```python
from build123d import *

# Parameters (mm, degrees)
BOSS_EXTRUDE2_DEPTH = 20
SKETCH2_R           = 1.5
CUT_EXTRUDE1_DEPTH  = 30


with BuildPart() as part:
    # Sketch1 → Boss-Extrude2 (new body)
    with BuildSketch(Plane.XY):
        with BuildLine():
            Line((-14, 17.3), (-26.4, 17.3))
            ThreePointArc((-26.4, 17.3), (-29.228427125, 18.471572875), (-30.4, 21.3))
            Line((-30.4, 21.3), (-30.4, 62.205522081))
            Line((-30.4, 62.205522081), (-27.4, 62.205522081))
            Line((-27.4, 62.205522081), (-27.4, 28.3))
            ThreePointArc((-27.4, 28.3), (-26.228427125, 25.471572875), (-23.4, 24.3))
            Line((-23.4, 24.3), (-3, 24.3))
            ThreePointArc((-3, 24.3), (-0.171572875, 23.128427125), (1, 20.3))
            Line((1, 20.3), (1, 9.949874371))
            ThreePointArc((1, 9.949874371), (6.708203932, -7.416198487), (-10, 0))
            Line((-10, 0), (-10, 13.3))
            ThreePointArc((-10, 13.3), (-11.171572875, 16.128427125), (-14, 17.3))
        make_face()
    extrude(amount=BOSS_EXTRUDE2_DEPTH)

    # Sketch2 → Cut-Extrude1 (cut)
    with BuildSketch(Plane.XY.offset(20)):
        Circle(SKETCH2_R)
    extrude(amount=-CUT_EXTRUDE1_DEPTH, mode=Mode.SUBTRACT)


solid = part.part
```
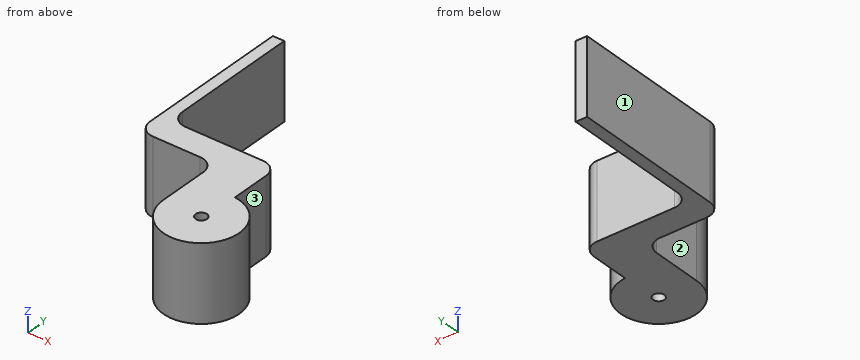
Design review of the part built by this model. Coordinates are the model's own, in mm. Face numbers are marked on the shaded views. A direction names the side the tool comes from. Coordinates: 2 decimals unless noted, no trailing zeros. Write each loop counter-clockwise with the first axis right and the second up, starting at its lowest first coordinate (ties: lowest second). Pieces come first, ordered by that corner, then holes. Notation, with made-up numbers: M -1.5,17 L 6.5,17 A26 cw 6.5,53 Z; hole C 8.25,50 d8. An arc over 180 degrees is marked long. Answer as a JSON object with one key per item and string values.
Item 1: Wall thickness on probe 1 along X at (y, z) = (46.5, 9.25); probe 2 along Y at (x, z) = (0, 13.25); probe 3 along Y at (x, z) = (-20.5, 3.75): over which ranges is each line inside the solid? List them lowest first.
Outcome:
{"probe 1": "-30.4 to -27.4", "probe 2": "-10 to -1.5, 1.5 to 22.95", "probe 3": "17.3 to 24.3"}
Item 2: Add section A-A, the plane z = 3. Give the boundary of the cut face in (x, y), and give its area (3 significant figures).
Outcome:
{"outline": "M -30.4,21.3 A4 ccw -26.4,17.3 L -14,17.3 A4 cw -10,13.3 L -10,0 A10 ccw long 1,9.95 L 1,20.3 A4 ccw -3,24.3 L -23.4,24.3 A4 cw -27.4,28.3 L -27.4,62.21 L -30.4,62.21 Z; hole C 0,0 d3", "area": "742 mm²"}
Item 3: Insertion check: pin 1 Ø6.5 at (y, z) = (8.5, 7) entering from -X; pin 2 Ø8 at (x, z) = (-2, 7.5) entering from -Y; pin 3 Ø10 at (y, z) = (38.5, 9.5) entering from +X; pin 4 Ø8 at (x, z) = (-26, 5.5) entering from -Y. Each pin has a flat end and moves straight along its axis. Give the tip position at first contact, or say it passes through.
Outcome:
{"pin 1": "x = -10", "pin 2": "y = -10", "pin 3": "x = -27.4", "pin 4": "y = 17.3"}
Item 4: Add section C-C, the plane y = 48. Give the boundary of the cut face in (x, z).
Outcome:
{"outline": "M -30.4,0 L -27.4,0 L -27.4,20 L -30.4,20 Z"}
Item 5: Machinability: for the marked faces 1, 2 and 3, which of the approach directions +Z, -Z, +X, -X, +Y, -Y give a long, thin tool a straight path to every point of the face, cutting with its end or side? Answer none if there is none.
Outcome:
{"face 1": "+Z, -Z, -X, +Y, -Y", "face 2": "+Z, -Z, -X, -Y", "face 3": "+Z, -Z, +X, +Y"}
Item 6: Add section B-B, the plane x = 0. Give the boundary of the cut face in (y, z), and give its area (3 significant figures).
Outcome:
{"outline": "M -10,0 L -1.5,0 L -1.5,20 L -10,20 Z; M 1.5,0 L 22.95,0 L 22.95,20 L 1.5,20 Z", "area": "599 mm²"}
Item 7: Add section D-D, the plane x = -21.5. Give the boundary of the cut face in (y, z).
Outcome:
{"outline": "M 17.3,0 L 24.3,0 L 24.3,20 L 17.3,20 Z"}
